Could you check a few things on this model? Use its own coordinates, in mm. A direction names the side the tool comes from. Coordinates: 2 decimals unless noted, no trailing zeros. Loops run counter-clockwise (first coordinate to the right, second up) from the corner with the lowest first, then second, coordinate; pieces in that order, holes last. Notation, with made-up numbers: (0.25, -24) - (30.25, -24) arc R25 ccw to (30.25, -12) - close; hole circle Ø6 at (29.25, -25). An arc over 180 degrees is marked (long way). Put each result on its own line as item: value. Start each with the question number.
```python
from build123d import *

# Parameters (mm, degrees)
BOSS_EXTRUDE2_DEPTH = 3
BOSS_EXTRUDE3_DEPTH = 50
FILLET3_R           = 1
SKETCH4_R           = 1.5
CUT_EXTRUDE1_DEPTH  = 40
SKETCH5_R           = 4.5
SKETCH5_W           = 40
SKETCH5_H           = 10
CUT_EXTRUDE2_DEPTH  = 10
FILLET4_R           = 2


with BuildPart() as part:
    # Sketch1 → Boss-Extrude2 (new body)
    with BuildSketch(Plane(origin=(0, 0, 0), x_dir=(1, 0, 0), z_dir=(0, 1, 0))):
        with BuildLine():
            Line((-36.64598461, 13.50127958), (43.35401539, 13.50127958))
            ThreePointArc((43.35401539, 13.50127958), (46.889549296, 12.036813486), (48.35401539, 8.50127958))
            Line((48.35401539, 8.50127958), (48.35401539, -11.49872042))
            ThreePointArc((48.35401539, -11.49872042), (46.889549296, -15.034254326), (43.35401539, -16.49872042))
            Line((43.35401539, -16.49872042), (-36.64598461, -16.49872042))
            ThreePointArc((-36.64598461, -16.49872042), (-40.181518516, -15.034254326), (-41.64598461, -11.49872042))
            Line((-41.64598461, -11.49872042), (-41.64598461, 8.50127958))
            ThreePointArc((-41.64598461, 8.50127958), (-40.181518516, 12.036813486), (-36.64598461, 13.50127958))
        make_face()
    extrude(amount=BOSS_EXTRUDE2_DEPTH)

    # Sketch3 → Boss-Extrude3 (add)
    with BuildSketch(Plane(origin=(0, 3, 0), x_dir=(1, 0, 0), z_dir=(0, 1, 0))):
        with BuildLine():
            Line((-36.64598461, -16.49872042), (43.35401539, -16.49872042))
            ThreePointArc((43.35401539, -16.49872042), (46.889549296, -15.034254326), (48.35401539, -11.49872042))
            Line((48.35401539, -11.49872042), (48.35401539, 8.50127958))
            ThreePointArc((48.35401539, 8.50127958), (46.889549296, 12.036813486), (43.35401539, 13.50127958))
            Line((43.35401539, 13.50127958), (-36.64598461, 13.50127958))
            ThreePointArc((-36.64598461, 13.50127958), (-40.181518516, 12.036813486), (-41.64598461, 8.50127958))
            Line((-41.64598461, 8.50127958), (-41.64598461, -11.49872042))
            ThreePointArc((-41.64598461, -11.49872042), (-40.181518516, -15.034254326), (-36.64598461, -16.49872042))
        make_face()
        with BuildLine():
            Line((-36.64598461, 5.50127958), (-36.64598461, -8.49872042))
            ThreePointArc((-36.64598461, -8.49872042), (-35.181518516, -12.034254326), (-31.64598461, -13.49872042))
            Line((-31.64598461, -13.49872042), (38.35401539, -13.49872042))
            ThreePointArc((38.35401539, -13.49872042), (41.889549296, -12.034254326), (43.35401539, -8.49872042))
            Line((43.35401539, -8.49872042), (43.35401539, 5.50127958))
            ThreePointArc((43.35401539, 5.50127958), (41.889549296, 9.036813486), (38.35401539, 10.50127958))
            Line((38.35401539, 10.50127958), (-31.64598461, 10.50127958))
            ThreePointArc((-31.64598461, 10.50127958), (-35.181518516, 9.036813486), (-36.64598461, 5.50127958))
        make_face(mode=Mode.SUBTRACT)
    extrude(amount=BOSS_EXTRUDE3_DEPTH)

    # Fillet3
    fillet3_edges = [part.edges().sort_by_distance(p)[0] for p in [
        (48.35401539, 0, 1.49872042),
        (46.889549296, 0, 15.034254326),
        (3.35401539, 0, 16.49872042),
        (-40.181518516, 0, 15.034254326),
        (-41.64598461, 0, 1.49872042),
        (-40.181518516, 0, -12.036813486),
        (3.35401539, 0, -13.50127958),
        (46.889549296, 0, -12.036813486),
    ]]
    fillet(fillet3_edges, radius=FILLET3_R)

    # Sketch4 → Cut-Extrude1 (cut)
    with BuildSketch(Plane(origin=(0, 53, 0), x_dir=(1, 0, 0), z_dir=(0, 1, 0))):
        with Locations(Location((-37.819946043, 9.867837779, 0), (0, 0, 270))):
            Circle(SKETCH4_R)
        with Locations(Location((-37.819946043, -12.865278618, 0), (0, 0, 90))):
            Circle(SKETCH4_R)
        with Locations(Location((44.527976823, -12.865278618, 0), (0, 0, 270))):
            Circle(SKETCH4_R)
        with Locations(Location((44.527976823, 9.867837779, 0), (0, 0, 90))):
            Circle(SKETCH4_R)
    extrude(amount=-CUT_EXTRUDE1_DEPTH, mode=Mode.SUBTRACT)

    # Sketch5 → Cut-Extrude2 (cut)
    with BuildSketch(Plane.XZ):
        with Locations(Location((33.20043836, 1.111101434, 0), (0, 0, 270))):
            Circle(SKETCH5_R)
        with Locations(Location((-26.79956164, 1.111101434, 0), (0, 0, 270))):
            Circle(SKETCH5_R)
        with Locations((3.20043836, 1.111101434)):
            Rectangle(SKETCH5_W, SKETCH5_H)
    extrude(amount=-CUT_EXTRUDE2_DEPTH, mode=Mode.SUBTRACT)

    # Fillet4
    fillet4_edges = [part.edges().sort_by_distance(p)[0] for p in [
        (3.20043836, 3, 6.111101434),
        (-16.79956164, 3, 1.111101434),
        (3.20043836, 3, -3.888898566),
        (23.20043836, 3, 1.111101434),
        (-26.79956164, 3, 5.611101434),
        (33.20043836, 3, 5.611101434),
        (41.889549296, 3, -9.036813486),
        (3.35401539, 3, -10.50127958),
        (-35.181518516, 3, -9.036813486),
        (-36.64598461, 3, 1.49872042),
        (-35.181518516, 3, 12.034254326),
        (3.35401539, 3, 13.49872042),
        (41.889549296, 3, 12.034254326),
        (43.35401539, 3, 1.49872042),
    ]]
    fillet(fillet4_edges, radius=FILLET4_R)


solid = part.part
```
(1) I want a section at C-C on z = -2.5. Count the separate pieces of the cut face and the enclosed holes in it, and give its area (3 significant figures).
(2) I want a section at D-D on y = 49. List the corners of the cut face in (x, z) for me, and give its area (3 significant figures).
(3) I want a section at B-B on x = 4. List the corners of the cut face in (y, z) for me, and give its area (3 significant figures).
(4) I need wall thicknesses on L1, parallel to X at y = 44.5, z = 8.5; L2, parallel to Z at x = -27.5, y = 38; L3, parallel to X at y = 35, z = 11.75. Which ranges of each line are inside material? Lowest first, please. Write a range as [from, to].
(5) I want a section at A-A on y = 11. List the corners of the cut face in (x, z) for me.
(6) Which directions (+Z, -Z, +X, -X, +Y, -Y) give clear straight access to the entire face, cutting with the end or side of a thin tool? Please do faces 5 (the cylindrical face through (23.77, 2.4, 1.21)), 6 (the flat face through (3, 53, 14)).
(7) If we mould it in two halves opening along Z, with no side actions, what happens to faces 1 (the cylindrical face through (46.85, 26.636, 15.073)), 2 (the cylindrical face through (2.86, 3.6, -9.93)), 3 (the flat face through (48.354, 27, 2)), 4 (the flat face through (3, 29, 13.499))? For each: pulls with the +Z half, pulls with the -Z half, needs draft (parallel to the pull), parting line crosses it, or undercut.
(8) For pin 1 Ø1.8 at (x, z) = (-37.82, -9.87) entering from +Y; pin 2 Ø3.5 at (x, z) = (-38, -10) entering from +Y; pin 3 Ø11.5 at (x, z) = (-26.8, 1.11) entering from +Y; pin 4 Ø10.5 at (x, z) = (33.2, 1.11) entering from +Y, each with a flat end and sliding along its axis, tell me the tip position at first contact or that it passes through.
Answer sheet:
1. separate pieces: 4
1. enclosed holes: 0
1. area: 612 mm^2
2. outline: (-41.65, -8.5) arc R5 ccw to (-36.65, -13.5) - (43.35, -13.5) arc R5 ccw to (48.35, -8.5) - (48.35, 11.5) arc R5 ccw to (43.35, 16.5) - (-36.65, 16.5) arc R5 ccw to (-41.65, 11.5) - close; hole circle Ø3 at (-37.82, -9.87); hole circle Ø3 at (-37.82, 12.87); hole (-36.65, -5.5) arc R5 ccw to (-31.65, -10.5) - (38.35, -10.5) arc R5 ccw to (43.35, -5.5) - (43.35, 8.5) arc R5 ccw to (38.35, 13.5) - (-31.65, 13.5) arc R5 ccw to (-36.65, 8.5) - close; hole circle Ø3 at (44.53, -9.87); hole circle Ø3 at (44.53, 12.87)
2. area: 752 mm^2
3. outline: (0, -12.5) arc R1 ccw to (1, -13.5) - (53, -13.5) - (53, -10.5) - (5, -10.5) arc R2 cw to (3, -8.5) - (3, -5.89) arc R2 ccw to (1, -3.89) - (0, -3.89) - close; (0, 6.11) - (1, 6.11) arc R2 ccw to (3, 8.11) - (3, 11.5) arc R2 cw to (5, 13.5) - (53, 13.5) - (53, 16.5) - (1, 16.5) arc R1 ccw to (0, 15.5) - close
3. area: 360 mm^2
4. L1: x = [-41.65, -36.65], [43.35, 48.35]
4. L2: z = [-13.5, -10.5], [13.5, 16.5]
4. L3: x = [-41.64, -38.82], [-36.82, -35.44], [42.15, 43.52], [45.53, 48.35]
5. outline: (-41.65, -8.5) arc R5 ccw to (-36.65, -13.5) - (43.35, -13.5) arc R5 ccw to (48.35, -8.5) - (48.35, 11.5) arc R5 ccw to (43.35, 16.5) - (-36.65, 16.5) arc R5 ccw to (-41.65, 11.5) - close; hole (-36.65, -5.5) arc R5 ccw to (-31.65, -10.5) - (38.35, -10.5) arc R5 ccw to (43.35, -5.5) - (43.35, 8.5) arc R5 ccw to (38.35, 13.5) - (-31.65, 13.5) arc R5 ccw to (-36.65, 8.5) - close
6. face 5: +Y
6. face 6: +Z, -Z, +X, -X, +Y
7. face 1: pulls with the +Z half
7. face 2: undercut
7. face 3: needs draft
7. face 4: undercut
8. pin 1: stops at y = 13
8. pin 2: stops at y = 53
8. pin 3: stops at y = 2.85
8. pin 4: stops at y = 2.56
